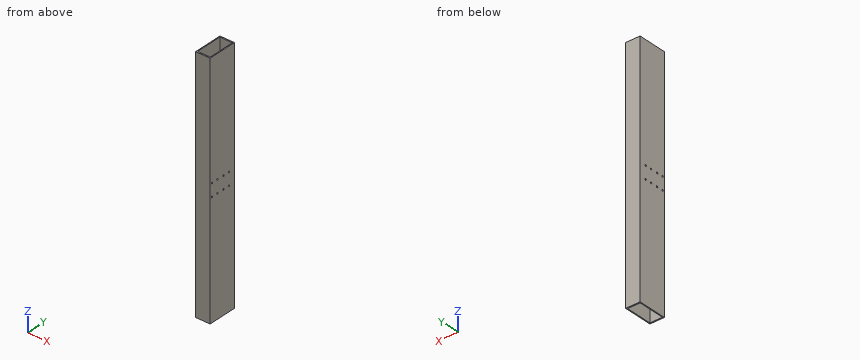
from build123d import *

# Parameters (mm, degrees)
SKETCH1_W                = 60
SKETCH1_H                = 120
SKETCH1_W_2              = 52
SKETCH1_H_2              = 110
F_7_0_7_DIAMETER_HOLE1_D = 7


with BuildPart() as part:
    # Sweep1: sweep along a curve in space
    with BuildLine() as sweep1_path:
        add(Edge.make_bspline(
            [(0, 0, -500), (0, 0, 500)],
            knots=[0, 0, 1, 1], degree=1))
    # Sketch1 → Sweep1 (sweep)
    with BuildSketch(Plane.XY):
        Rectangle(SKETCH1_W, SKETCH1_H)
        Rectangle(SKETCH1_W_2, SKETCH1_H_2, mode=Mode.SUBTRACT)
    sweep(path=sweep1_path.line)

    # Ø7.0 (7) Diameter Hole1 (through all)
    with Locations(Plane(origin=(30, 0, 0), x_dir=(0, 0, -1), z_dir=(1, 0, 0))):
        with Locations((26, 33), (26, 6), (26, -24), (26, -51)):
            f_7_0_7_diameter_hole1 = Hole(F_7_0_7_DIAMETER_HOLE1_D / 2)

    # Mirror1: Ø7.0 (7) Diameter Hole1 across plane
    add(f_7_0_7_diameter_hole1.mirror(Plane.XY), mode=Mode.SUBTRACT)


solid = part.part
The model under review builds one solid part; all positions refer to its coordinate system, in mm. Give positions to 0.01 mm unless a question says otherwise; leave off trailing zeros. Order: outer loops, then holes, each group sorted by start corner. A loop starts at its lowest first (then second) coordinate and runs counter-clockwise, first axis right, second up. Notation, with made-up numbers: M 29,44 L 51,44 A11 ccw 51,61 Z; hole C 45.25,29.25 d10. An arc over 180 degrees is marked long. Use one line per item in the form item = value. Start each with the question number.
Item 1: Insertion check: pin 1 Ø11 at (y, z) = (-24, 26) entering from +X; pin 2 Ø4 at (y, z) = (33, 26) entering from -X. Each pin has a flat end and moves straight along its axis. Give the tip position at first contact, or say it passes through.
Item 2: We need section A-A on x = 11. Give the boundary of the cut face in (y, z), plus the area to 4 significant figures.
Item 3: We need section B-B on z = 56.5. Give the boundary of the cut face in (x, y), plus the area to 3 significant figures.
Item 4: To check wall thickness, follow line 1 along Y through (x, z) = (-27, -26); line 2 along X through (y, z) = (-54, 424.5); line 3 along Y through (x, z) = (9, 49.5). State the ranges of each line that lie inside material, in increasing order. Write a range as from..to.
Completed:
q1.pin_1 = 30
q1.pin_2 = through
q2.outline = M -60,-500 L -55,-500 L -55,500 L -60,500 Z; M 55,-500 L 60,-500 L 60,500 L 55,500 Z
q2.area = 10,000 mm²
q3.outline = M -30,-60 L 30,-60 L 30,60 L -30,60 Z; hole M -26,-55 L 26,-55 L 26,55 L -26,55 Z
q3.area = 1,480 mm²
q4.line_1 = -60..-54.5, -47.5..-27.5, -20.5..2.5, 9.5..29.5, 36.5..60
q4.line_2 = -30..-26, 26..30
q4.line_3 = -60..-55, 55..60
